The listing builds one solid part. Answer for the finished solid, in the listing's coordinates (mm). A direction names the side the tool comes from. Coordinates: 2 decimals unless noted, no trailing zeros. Write each loop counter-clockwise with the first axis right and the second up, starting at its lowest first coordinate (ties: lowest second). Pieces come first, ordered by that corner, then holes.
```python
from build123d import *

# Parameters (mm, degrees)
SKETCH1_W           = 147.22869713
SKETCH1_H           = 40.463516098
BOSS_EXTRUDE1_DEPTH = 76.2
SHELL1_T            = -2.54
SKETCH2_W           = 122.174
SKETCH2_H           = 7.62
CUT_EXTRUDE1_DEPTH  = 2.54


with BuildPart() as part:
    # Sketch1 → Boss-Extrude1 (new body)
    with BuildSketch(Plane(origin=(0, 0, 0), x_dir=(1, 0, 0), z_dir=(0, 1, 0))):
        Rectangle(SKETCH1_W, SKETCH1_H)
    extrude(amount=BOSS_EXTRUDE1_DEPTH)

    # Shell1
    shell1_openings = [part.faces().sort_by_distance(p)[0] for p in [
        (0, 0, 0),
    ]]
    offset(amount=SHELL1_T, openings=shell1_openings, kind=Kind.INTERSECTION)

    # Sketch2 → Cut-Extrude1 (cut)
    with BuildSketch(Plane(origin=(0, 76.2, 0), x_dir=(1, 0, 0), z_dir=(0, 1, 0))):
        Rectangle(SKETCH2_W, SKETCH2_H)
    extrude(amount=-CUT_EXTRUDE1_DEPTH, mode=Mode.SUBTRACT)


solid = part.part
```
(1) Find the intervals of material crossed by probe 1 along Z at (x, y) = (25, 17); probe 2 along X at (y, z) = (60.5, -4.5); probe 3 along Y at (x, z) = (-2, 15), in increasing order.
(2) Section C-C, the plane y = 7 is taken. Write down the section's boundary in (x, z), plus the area to 3 significant figures.
(3) Which of the six approach directions +Z, -Z, +X, -X, +Y, -Y give full straight-line access (tool end or side, diameter ignored) to faces 1 (the flat face through (-1, 38, 20.232)), 2 (the flat face through (-71.074, 36, 0))?
(4) Section D-D, the plane x = -63.5 is taken. Write down the section's boundary in (y, z).
(5) For a pull along X with two mould halves and no side action, classify faces 3 (the flat face through (-1, 36, -17.692)), 4 (the flat face through (-1, 73.66, -4)), 5 (the flat face through (-11, 0, 18)), 6 (the flat face through (73.614, 38, 0)) as pulls with the +X half, pulls with the -X half, needs draft (parallel to the pull), parting line crosses it, or undercut.
(6) Section A-A, the plane x = -10 is taken. Write down the section's boundary in (y, z), plus the area to 3 significant figures.
(7) Section B-B, the plane z = -2 is taken. Write down the section's boundary in (x, y).
Solution:
1. probe 1: z = -20.23 to -17.69, 17.69 to 20.23
1. probe 2: x = -73.61 to -71.07, 71.07 to 73.61
1. probe 3: y = 73.66 to 76.2
2. outline: (-73.61, -20.23) - (73.61, -20.23) - (73.61, 20.23) - (-73.61, 20.23) - close; hole (-71.07, -17.69) - (71.07, -17.69) - (71.07, 17.69) - (-71.07, 17.69) - close
2. area: 928 mm2
3. face 1: +Z, +X, -X, +Y, -Y
3. face 2: -Y
4. outline: (0, -20.23) - (76.2, -20.23) - (76.2, 20.23) - (0, 20.23) - (0, 17.69) - (73.66, 17.69) - (73.66, -17.69) - (0, -17.69) - close
5. face 3: undercut
5. face 4: undercut
5. face 5: needs draft
5. face 6: pulls with the +X half
6. outline: (0, -20.23) - (76.2, -20.23) - (76.2, -3.81) - (73.66, -3.81) - (73.66, -17.69) - (0, -17.69) - close; (0, 17.69) - (73.66, 17.69) - (73.66, 3.81) - (76.2, 3.81) - (76.2, 20.23) - (0, 20.23) - close
6. area: 458 mm2
7. outline: (-73.61, 0) - (-71.07, 0) - (-71.07, 73.66) - (-61.09, 73.66) - (-61.09, 76.2) - (-73.61, 76.2) - close; (61.09, 73.66) - (71.07, 73.66) - (71.07, 0) - (73.61, 0) - (73.61, 76.2) - (61.09, 76.2) - close
